The model under review builds one solid part; all positions refer to its coordinate system, in mm. Round coordinates to 2 decimals unless told otherwise and drop trailing zeros. Order: outer loops, then holes, each group sorted by start corner. A loop starts at its lowest first (then second) coordinate and runs counter-clockwise, first axis right, second up.
1) Consider section B-B (y = 47). Give the boundary of the cut face in (x, z) (3 decimals).
2) Consider section D-D (z = 2.35). Give the number of separate pieces and of enclosed holes in the cut face, then the cut area to 3 significant figures.
3) Consider section C-C (y = -184). Give the boundary of the cut face in (x, z) (3 decimals), then the cut area to 3 significant figures.
4) To check wall thickness, follow L1, parallel to X at y = 44, z = 1.3; L2, parallel to X at y = -231, z = 2.95; L3, parallel to Y at x = -4, z = 3.55. State the ranges of each line that lie inside material, in increasing order.
5) Consider section A-A (x = 33.5). Give the boundary of the cut face in (y, z) (3 decimals), then the cut area to 4 significant figures.
6) Clearance check with flat-ended pins moving along their axes: P1, Ø0.8, axis at x = -61.5, z = 2.5, coming from the +Y side; P2, Ø3, axis at x = 179.06, y = 67.81, coming from the +Z side; P3, Ø1.6, axis at x = -61.5, z = 2.5, coming from the -Y side. State where each tip first meets the part, or that it passes through.
Autodesk Inventor part; units mm, degrees
ref_plane "YZ Plane" through (0, 0, 0) normal (1, 0, 0) x (0, 1, 0)
ref_plane "XZ Plane" through (0, 0, 0) normal (0, 1, 0) x (-1, 0, 0)
ref_plane "XY Plane" through (0, 0, 0) normal (0, 0, 1) x (1, 0, 0)
sketch "Sketch3" plane through (0, 0, 0) normal (0, 0, 1) x (1, 0, 0)
  line L0 (181.0574, -229.1936) -> (181.0574, -225.1936)
  line L1 (181.0574, -225.1936) -> (182.5574, -225.1936)
  line L2 (182.5574, -225.1936) -> (182.5574, -229.1936)
  line L3 (182.5574, -229.1936) -> (181.0574, -229.1936)
  line L4 (171.5574, -229.1936) -> (171.5574, -225.1936)
  line L5 (171.5574, -225.1936) -> (173.0574, -225.1936)
  line L6 (173.0574, -225.1936) -> (173.0574, -229.1936)
  line L7 (173.0574, -229.1936) -> (171.5574, -229.1936)
  circle A0 centre (179.0574, -242.1936) radius 2.5
  line L8 (112.0574, -234.1936) -> (112.0574, -194.1936)
  line L9 (112.0574, -194.1936) -> (147.0574, -194.1936)
  line L10 (147.0574, -194.1936) -> (147.0574, -234.1936)
  line L11 (147.0574, -234.1936) -> (112.0574, -234.1936)
  line L12 (181.0574, 54.8064) -> (181.0574, 50.8064)
  line L13 (182.5574, 54.8064) -> (181.0574, 54.8064)
  line L14 (182.5574, 50.8064) -> (182.5574, 54.8064)
  line L15 (181.0574, 50.8064) -> (182.5574, 50.8064)
  line L16 (171.5574, 54.8064) -> (171.5574, 50.8064)
  line L17 (173.0574, 54.8064) -> (171.5574, 54.8064)
  line L18 (173.0574, 50.8064) -> (173.0574, 54.8064)
  line L19 (171.5574, 50.8064) -> (173.0574, 50.8064)
  circle A1 centre (179.0574, 67.8064) radius 2.5
  line L20 (112.0574, 59.8064) -> (112.0574, 19.8064)
  line L21 (147.0574, 59.8064) -> (112.0574, 59.8064)
  line L22 (147.0574, 19.8064) -> (147.0574, 59.8064)
  line L23 (112.0574, 19.8064) -> (147.0574, 19.8064)
  line L24 (-60.9426, -229.1936) -> (-60.9426, -225.1936)
  line L25 (-62.4426, -229.1936) -> (-60.9426, -229.1936)
  line L26 (-62.4426, -225.1936) -> (-62.4426, -229.1936)
  line L27 (-60.9426, -225.1936) -> (-62.4426, -225.1936)
  line L28 (-51.4426, -229.1936) -> (-51.4426, -225.1936)
  line L29 (-52.9426, -229.1936) -> (-51.4426, -229.1936)
  line L30 (-52.9426, -225.1936) -> (-52.9426, -229.1936)
  line L31 (-51.4426, -225.1936) -> (-52.9426, -225.1936)
  circle A2 centre (-58.9426, -242.1936) radius 2.5
  line L32 (8.0574, -234.1936) -> (8.0574, -194.1936)
  line L33 (-26.9426, -234.1936) -> (8.0574, -234.1936)
  line L34 (-26.9426, -194.1936) -> (-26.9426, -234.1936)
  line L35 (8.0574, -194.1936) -> (-26.9426, -194.1936)
  arc A3 (-66.9426, 49.8064) -> (-64.9426, 47.8064) centre (-64.9426, 49.8064) ccw
  line L36 (-64.9426, 47.8064) -> (-58.9426, 47.8064)
  line L37 (-58.9426, 47.8064) -> (-58.9426, 57.8064)
  line L38 (-58.9426, 57.8064) -> (-54.9426, 57.8064)
  line L39 (-54.9426, 57.8064) -> (-54.9426, 47.8064)
  line L40 (-54.9426, 47.8064) -> (-48.9426, 47.8064)
  arc A4 (-46.9426, 45.8064) -> (-48.9426, 47.8064) centre (-48.9426, 45.8064) ccw
  line L41 (-46.9426, 45.8064) -> (-46.9426, -220.1936)
  arc A5 (-48.9426, -222.1936) -> (-46.9426, -220.1936) centre (-48.9426, -220.1936) ccw
  line L42 (-54.9426, -222.1936) -> (-48.9426, -222.1936)
  line L43 (-54.9426, -232.1936) -> (-54.9426, -222.1936)
  line L44 (-58.9426, -232.1936) -> (-54.9426, -232.1936)
  line L45 (-58.9426, -222.1936) -> (-58.9426, -232.1936)
  line L46 (-64.9426, -222.1936) -> (-58.9426, -222.1936)
  arc A6 (-64.9426, -222.1936) -> (-66.9426, -224.1936) centre (-64.9426, -224.1936) ccw
  line L47 (-66.9426, -242.1936) -> (-66.9426, -224.1936)
  arc A7 (-66.9426, -242.1936) -> (-58.9426, -250.1936) centre (-58.9426, -242.1936) ccw
  line L48 (179.0574, -250.1936) -> (-58.9426, -250.1936)
  arc A8 (179.0574, -250.1936) -> (187.0574, -242.1936) centre (179.0574, -242.1936) ccw
  line L49 (187.0574, -242.1936) -> (187.0574, -224.1936)
  arc A9 (187.0574, -224.1936) -> (185.0574, -222.1936) centre (185.0574, -224.1936) ccw
  line L50 (185.0574, -222.1936) -> (179.0574, -222.1936)
  line L51 (179.0574, -222.1936) -> (179.0574, -232.1936)
  line L52 (179.0574, -232.1936) -> (175.0574, -232.1936)
  line L53 (175.0574, -232.1936) -> (175.0574, -222.1936)
  line L54 (175.0574, -222.1936) -> (169.0574, -222.1936)
  arc A10 (167.0574, -220.1936) -> (169.0574, -222.1936) centre (169.0574, -220.1936) ccw
  line L55 (167.0574, -220.1936) -> (167.0574, 45.8064)
  arc A11 (169.0574, 47.8064) -> (167.0574, 45.8064) centre (169.0574, 45.8064) ccw
  line L56 (175.0574, 47.8064) -> (169.0574, 47.8064)
  line L57 (175.0574, 57.8064) -> (175.0574, 47.8064)
  line L58 (179.0574, 57.8064) -> (175.0574, 57.8064)
  line L59 (179.0574, 47.8064) -> (179.0574, 57.8064)
  line L60 (185.0574, 47.8064) -> (179.0574, 47.8064)
  arc A12 (185.0574, 47.8064) -> (187.0574, 49.8064) centre (185.0574, 49.8064) ccw
  line L61 (187.0574, 67.8064) -> (187.0574, 49.8064)
  arc A13 (187.0574, 67.8064) -> (179.0574, 75.8064) centre (179.0574, 67.8064) ccw
  line L62 (-58.9426, 75.8064) -> (179.0574, 75.8064)
  arc A14 (-58.9426, 75.8064) -> (-66.9426, 67.8064) centre (-58.9426, 67.8064) ccw
  line L63 (-66.9426, 67.8064) -> (-66.9426, 49.8064)
  line L64 (8.0574, 59.8064) -> (8.0574, 19.8064)
  line L65 (8.0574, 19.8064) -> (-26.9426, 19.8064)
  line L66 (-26.9426, 19.8064) -> (-26.9426, 59.8064)
  line L67 (-26.9426, 59.8064) -> (8.0574, 59.8064)
  circle A15 centre (-58.9426, 67.8064) radius 2.5
  line L68 (-51.4426, 54.8064) -> (-51.4426, 50.8064)
  line L69 (-51.4426, 50.8064) -> (-52.9426, 50.8064)
  line L70 (-52.9426, 50.8064) -> (-52.9426, 54.8064)
  line L71 (-52.9426, 54.8064) -> (-51.4426, 54.8064)
  line L72 (-60.9426, 54.8064) -> (-60.9426, 50.8064)
  line L73 (-60.9426, 50.8064) -> (-62.4426, 50.8064)
  line L74 (-62.4426, 50.8064) -> (-62.4426, 54.8064)
  line L75 (-62.4426, 54.8064) -> (-60.9426, 54.8064)
  line L76 (-66.9426, 49.8064) -> (-66.9426, -224.1936)
  line L77 (187.0574, -224.1936) -> (187.0574, 49.8064)
  line L78 (-26.9426, 39.8064) -> (8.0574, 39.8064)
  line L79 (112.0574, 39.8064) -> (147.0574, 39.8064)
  line L80 (-26.9426, -214.1936) -> (8.0574, -214.1936)
  line L81 (112.0574, -214.1936) -> (147.0574, -214.1936)
  line L82 (65.0574, 54.8064) -> (65.0574, 30.8064)
  arc A16 (65.0574, 30.8064) -> (70.0574, 25.8064) centre (70.0574, 30.8064) ccw
  line L83 (70.0574, 25.8064) -> (72.5574, 25.8064)
  line L84 (72.5574, 25.8064) -> (72.5574, 13.3064)
  arc A17 (47.5574, 13.3064) -> (72.5574, 13.3064) centre (60.0574, 13.3064) ccw
  line L85 (47.5574, 13.3064) -> (47.5574, 25.8064)
  line L86 (47.5574, 25.8064) -> (50.0574, 25.8064)
  arc A18 (50.0574, 25.8064) -> (55.0574, 30.8064) centre (50.0574, 30.8064) ccw
  line L87 (55.0574, 30.8064) -> (55.0574, 54.8064)
  arc A19 (65.0574, 54.8064) -> (55.0574, 54.8064) centre (60.0574, 54.8064) ccw
  point P0 (0, 0)
extrude "Extrusion3" add sketch "Sketch3" along normal blind 5.715 contours L8 L9 L10 L81 | L79 L22 L23 L20 | L80 L34 L35 L32 | L63 A14 L62 A13 L61 A12 L60 L59 L58 L57 L56 A11 L55 A10 L54 L53 L52 L51 L50 A9 L49 A8 L48 A7 L47 A6 L46 L45 L44 L43 L42 A5 L41 A4 L40 L39 L38 L37 L36 A3 | A3 L36 L37 L38 L39 L40 A4 L41 A5 L42 L43 L44 L45 L46 A6 L76 | L77 A9 L50 L51 L52 L53 L54 A10 L55 A11 L56 L57 L58 L59 L60 A12 | L64 L65 L66 L78 | L82 A16 L83 L84 A17 L85 L86 A18 L87 A19
sketch "Sketch4" plane through (0, 0, 5.715) normal (0, 0, 1) x (1, 0, 0)
  line L0 (187.0574, -242.1936) -> (187.0574, 67.8064)
  line L1 (179.0574, 75.8064) -> (-58.9426, 75.8064)
  line L2 (-52.9426, 25.8064) -> (173.0574, 25.8064)
  line L3 (173.0574, 25.8064) -> (173.0574, -200.1936)
  line L4 (173.0574, -200.1936) -> (-52.9426, -200.1936)
  line L5 (-52.9426, -200.1936) -> (-52.9426, 25.8064)
  point P0 (0, 0)
  point P1 (60.0574, 25.8064)
  point P2 (60.0574, 75.8064)
  point P3 (173.0574, -87.1936)
  point P4 (187.0574, -87.1936)
  dimension "d8" = 226
extrude "Extrusion4" cut sketch "Sketch4" against normal through all
sketch "Sketch5" plane through (0, 0, 5.715) normal (0, 0, 1) x (1, 0, 0)
  line L0 (-52.9426, 25.8064) -> (173.0574, 25.8064)
  line L1 (147.0574, 39.8064) -> (112.0574, 39.8064)
  line L2 (179.0574, 75.8064) -> (-58.9426, 75.8064)
  line L3 (55.0574, 25.8064) -> (55.0574, 59.8064)
  line L4 (55.0574, 59.8064) -> (65.0574, 59.8064)
  line L5 (65.0574, 59.8064) -> (65.0574, 25.8064)
  point P0 (0, 0)
  point P1 (60.0574, 59.8064)
  point P2 (60.0574, 25.8064)
  dimension "d12" = 10
  dimension "d15" = 20
extrude "Extrusion5" cut sketch "Sketch5" against normal through all
fillet "Fillet1" radius 5 4 edges at (55.0574, 25.8064, 2.8575) (55.0574, 59.8064, 2.8575) (65.0574, 59.8064, 2.8575) (65.0574, 25.8064, 2.8575)
properties part number "BED PLATE TOP"
Answer below:
1. outline: (-66.943, 0) - (-26.943, 0) - (-26.943, 5.715) - (-66.943, 5.715) - close; (8.057, 0) - (55.057, 0) - (55.057, 5.715) - (8.057, 5.715) - close; (65.057, 0) - (112.057, 0) - (112.057, 5.715) - (65.057, 5.715) - close; (147.057, 0) - (187.057, 0) - (187.057, 5.715) - (147.057, 5.715) - close
2. separate pieces: 1
2. enclosed holes: 17
2. area: 28,400 mm2
3. outline: (-66.943, 0) - (-52.943, 0) - (-52.943, 5.715) - (-66.943, 5.715) - close; (173.057, 0) - (187.057, 0) - (187.057, 5.715) - (173.057, 5.715) - close
3. area: 160 mm2
4. L1: x = -66.94 to -26.94, 8.06 to 55.06, 65.06 to 112.06, 147.06 to 187.06
4. L2: x = -66.94 to -26.94, 8.06 to 112.06, 147.06 to 187.06
4. L3: y = -250.19 to -234.19, -214.19 to -200.19, 25.81 to 39.81, 59.81 to 75.81
5. outline: (-250.194, 0) - (-200.194, 0) - (-200.194, 5.715) - (-250.194, 5.715) - close; (25.806, 0) - (75.806, 0) - (75.806, 5.715) - (25.806, 5.715) - close
5. area: 571.5 mm2
6. P1: stops at y = 75.51
6. P2: passes through
6. P3: stops at y = -250
